```python
from build123d import *

# Parameters (mm, degrees)
BOSS_EXTRUDE1_DEPTH = 200


with BuildPart() as part:
    # Sketch1 → Boss-Extrude1 (new body)
    with BuildSketch(Plane.XY):
        Polygon((60, -7.5), (35.9, -7.5), (35.9, -5.7), (40, -5.7), (40, -3.9), (37.900227313, 0.5), (25.900227313, 0.5), (24, -3.989786353), (24, -5.7), (28.1, -5.7), (28.1, -7.5), (3.9, -7.5), (3.9, -5.7), (8, -5.7), (8, -3.9), (5.900227313, 0.5), (-6.099772687, 0.5), (-8, -3.989786353), (-8, -5.7), (-3.9, -5.7), (-3.9, -7.5), (-28.1, -7.5), (-28.1, -5.7), (-24, -5.7), (-24, -3.9), (-26.099772687, 0.5), (-38.099772687, 0.5), (-40, -3.989786353), (-40, -5.7), (-35.9, -5.7), (-35.9, -7.5), (-60, -7.5), (-60, 7.5), (-51.9, 7.5), (-51.9, 5.7), (-56, 5.7), (-56, 3.9), (-54, -0.5), (-42, -0.5), (-40, 3.9), (-40, 5.7), (-44.1, 5.7), (-44.1, 7.5), (-19.9, 7.5), (-19.9, 5.7), (-24, 5.7), (-24, 3.9), (-22, -0.5), (-10, -0.5), (-8, 3.9), (-8, 5.7), (-12.1, 5.7), (-12.1, 7.5), (12.1, 7.5), (12.1, 5.7), (8, 5.7), (8, 3.9), (10, -0.5), (22, -0.5), (24, 3.9), (24, 5.7), (19.9, 5.7), (19.9, 7.5), (44.1, 7.5), (44.1, 5.7), (40, 5.7), (40, 3.9), (42, -0.5), (54, -0.5), (56, 3.9), (56, 5.7), (51.9, 5.7), (51.9, 7.5), (60, 7.5), align=None)
    extrude(amount=BOSS_EXTRUDE1_DEPTH)


solid = part.part
```
Verification items for the finished model (mm, model axes). Give positions to 0.01 mm unless a question says otherwise; leave off trailing zeros. Order: outer loops, then holes, each group sorted by start corner. A loop starts at its lowest first (then second) coordinate and runs counter-clockwise, first axis right, second up. Notation, with made-up numbers: M 44,68.5 L 48,68.5 A13 cw 48,80.5 Z; hole C 4,21 d9. An arc over 180 degrees is marked long. Return JSON: item names as keys, results as strings. Group by question number.
1) Scan lines: line 1 (X direction, y = -5, z = 156); line 2 (X direction, y = 6.5, z = 90); line 3 (X direction, y = -5.75, z = 43.5). Record each from-to range of solid material in increasing order.
2) Section check A-A on x = -50. Record the cut outline in (y, z).
3) Mould release check, pull along Y, two halves, no side actions. Record for faces 1 (the face through (-48, -7.5, 99)), 2 (the face through (54, 5.7, 99)): pulls with the +Y half, pulls with the -Y half, needs draft (parallel to the pull), parting line crosses it, or undercut.
4) Go/stop test with a flat-tipped pin: pin 1 Ø1 at (x, z) = (-34, 36) entering from -Y. Record where the tip stops, or that it passes through.
Answer block:
{
 "1": {"line 1": "x = -60 to -40, -24 to -8, 8 to 24, 40 to 60", "line 2": "x = -60 to -51.9, -44.1 to -19.9, -12.1 to 12.1, 19.9 to 44.1, 51.9 to 60", "line 3": "x = -60 to -35.9, -28.1 to -3.9, 3.9 to 28.1, 35.9 to 60"},
 "2": {"outline": "M -7.5,0 L -0.5,0 L -0.5,200 L -7.5,200 Z"},
 "3": {"face 1": "pulls with the -Y half", "face 2": "undercut"},
 "4": {"pin 1": "stops at y = 0.5"}
}
